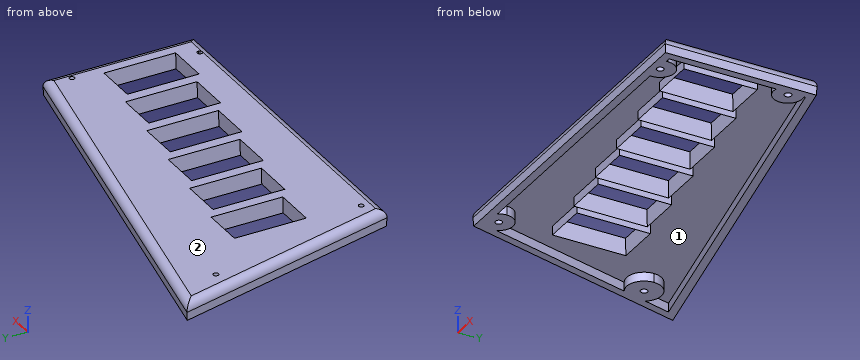
from build123d import *

# Parameters (mm, degrees)
F0_R        = 1.75
F0_W        = 22
F0_H        = 37
F1_DEPTH    = 8.5
F1_TAPER    = -3
F2_DEPTH    = 4.5
F3_T1_DEPTH = 142.1271805444
F3_T3_DEPTH = 228.1816697632
F3_T5_DEPTH = 194.8691049092
F3_T7_DEPTH = 97.8862114568


# Not quite as in the source:
# - a fillet or chamfer that OpenCascade refuses, or shapes differently, is made with other operations: its cross-section is extruded or revolved along the edge and cut away or added


with BuildPart() as f1:
    # F0 (on Top) → F1 (new body)
    with BuildSketch(Plane.XY):
        with BuildLine():
            ThreePointArc((-85.7353818111, -46.3140564233), (-82.1998275149, -55.281625252), (-72.882363358, -52.811342563))
            Line((-72.882363358, -52.811342563), (-84.115426434, -52.811342563))
            Line((-84.115426434, -52.811342563), (-85.7353818111, -46.3140564233))
        make_face()
        with BuildLine():
            Line((-84.115426434, -52.811342563), (-72.882363358, -52.811342563))
            ThreePointArc((-72.882363358, -52.811342563), (-71.9863977223, -50.8998795502), (-71.6790566692, -48.811342563))
            ThreePointArc((-71.6790566692, -48.811342563), (-77.6608605642, -41.6731229923), (-85.7353818111, -46.3140564233))
            Line((-85.7353818111, -46.3140564233), (-84.115426434, -52.811342563))
        make_face()
        with Locations((-78.9290566692, -48.811342563)):
            Circle(F0_R, mode=Mode.SUBTRACT)
        with BuildLine():
            ThreePointArc((73.5070839924, -52.811342563), (72.0709433308, -53.561342563), (70.6348026691, -52.811342563))
            Line((70.6348026691, -52.811342563), (64.8902400226, -52.811342563))
            ThreePointArc((64.8902400226, -52.811342563), (65.5417323383, -54.9628348787), (66.8209433308, -56.811342563))
            Line((66.8209433308, -56.811342563), (77.3209433308, -56.811342563))
            ThreePointArc((77.3209433308, -56.811342563), (78.6001543232, -54.9628348787), (79.2516466389, -52.811342563))
            Line((79.2516466389, -52.811342563), (73.5070839924, -52.811342563))
        make_face()
        with BuildLine():
            ThreePointArc((70.6348026691, -52.811342563), (71.5468947442, -50.1416500527), (73.8209433308, -51.811342563))
            ThreePointArc((73.8209433308, -51.811342563), (73.7406358411, -52.3353911496), (73.5070839924, -52.811342563))
            Line((73.5070839924, -52.811342563), (79.2516466389, -52.811342563))
            ThreePointArc((79.2516466389, -52.811342563), (79.3035984098, -52.3125416331), (79.3209433308, -51.811342563))
            ThreePointArc((79.3209433308, -51.811342563), (71.5697442607, -44.578687484), (64.8902400226, -52.811342563))
            Line((64.8902400226, -52.811342563), (70.6348026691, -52.811342563))
        make_face()
        with BuildLine():
            ThreePointArc((81.75943106, 15.1902968563), (72.6280630891, 8.188657437), (81.75943106, 1.1870180177))
            Line((81.75943106, 1.1870180177), (81.75943106, 15.1902968563))
        make_face()
        with Locations((79.8780630891, 8.188657437)):
            Circle(F0_R, mode=Mode.SUBTRACT)
        with BuildLine():
            Line((81.75943106, 15.1902968563), (81.75943106, 1.1870180177))
            ThreePointArc((81.75943106, 1.1870180177), (83.9978435057, 2.2229295418), (85.75943106, 3.9493165931))
            Line((85.75943106, 3.9493165931), (85.75943106, 12.4279982809))
            ThreePointArc((85.75943106, 12.4279982809), (83.9978435057, 14.1543853322), (81.75943106, 15.1902968563))
        make_face()
        with BuildLine():
            Line((-107.4844802754, 40.9168130189), (-104.4029422618, 28.5574391079))
            ThreePointArc((-104.4029422618, 28.5574391079), (-95.700189339, 28.6381178265), (-91.3719369109, 36.188657437))
            ThreePointArc((-91.3719369109, 36.188657437), (-97.6581749945, 44.5846313066), (-107.4844802754, 40.9168130189))
        make_face()
        with Locations((-100.1219369109, 36.188657437)):
            Circle(F0_R, mode=Mode.SUBTRACT)
        with BuildLine():
            ThreePointArc((-107.4844802754, 40.9168130189), (-108.6120245158, 34.0718408505), (-104.4029422618, 28.5574391079))
            Line((-104.4029422618, 28.5574391079), (-107.4844802754, 40.9168130189))
        make_face()
        with BuildLine():
            ThreePointArc((66.8209433308, -56.811342563), (65.5417323383, -54.9628348787), (64.8902400226, -52.811342563))
            Line((64.8902400226, -52.811342563), (-72.882363358, -52.811342563))
            ThreePointArc((-72.882363358, -52.811342563), (-82.1998275149, -55.281625252), (-85.7353818111, -46.3140564233))
            Line((-85.7353818111, -46.3140564233), (-104.4029422618, 28.5574391079))
            ThreePointArc((-104.4029422618, 28.5574391079), (-108.6120245158, 34.0718408505), (-107.4844802754, 40.9168130189))
            Line((-107.4844802754, 40.9168130189), (-110.8617073408, 54.4621309411))
            Line((-110.8617073408, 54.4621309411), (81.75943106, 15.9099091088))
            Line((81.75943106, 15.9099091088), (81.75943106, 15.1902968563))
            ThreePointArc((81.75943106, 15.1902968563), (83.9978435057, 14.1543853322), (85.75943106, 12.4279982809))
            Line((85.75943106, 12.4279982809), (85.75943106, 19.188657437))
            Line((85.75943106, 19.188657437), (-116.2711964119, 59.6241445901))
            Line((-116.2711964119, 59.6241445901), (-87.24056894, -56.811342563))
            Line((-87.24056894, -56.811342563), (66.8209433308, -56.811342563))
        make_face()
        with BuildLine():
            Line((81.75943106, -52.811342563), (79.2516466389, -52.811342563))
            ThreePointArc((79.2516466389, -52.811342563), (78.6001543232, -54.9628348787), (77.3209433308, -56.811342563))
            Line((77.3209433308, -56.811342563), (85.75943106, -56.811342563))
            Line((85.75943106, -56.811342563), (85.75943106, 3.9493165931))
            ThreePointArc((85.75943106, 3.9493165931), (83.9978435057, 2.2229295418), (81.75943106, 1.1870180177))
            Line((81.75943106, 1.1870180177), (81.75943106, -52.811342563))
        make_face()
        with BuildLine():
            Line((-72.882363358, -52.811342563), (64.8902400226, -52.811342563))
            ThreePointArc((64.8902400226, -52.811342563), (71.5697442607, -44.578687484), (79.3209433308, -51.811342563))
            ThreePointArc((79.3209433308, -51.811342563), (79.3035984098, -52.3125416331), (79.2516466389, -52.811342563))
            Line((79.2516466389, -52.811342563), (81.75943106, -52.811342563))
            Line((81.75943106, -52.811342563), (81.75943106, 1.1870180177))
            ThreePointArc((81.75943106, 1.1870180177), (72.6280630891, 8.188657437), (81.75943106, 15.1902968563))
            Line((81.75943106, 15.1902968563), (81.75943106, 15.9099091088))
            Line((81.75943106, 15.9099091088), (-110.8617073408, 54.4621309411))
            Line((-110.8617073408, 54.4621309411), (-107.4844802754, 40.9168130189))
            ThreePointArc((-107.4844802754, 40.9168130189), (-97.6581749945, 44.5846313066), (-91.3719369109, 36.188657437))
            ThreePointArc((-91.3719369109, 36.188657437), (-95.700189339, 28.6381178265), (-104.4029422618, 28.5574391079))
            Line((-104.4029422618, 28.5574391079), (-85.7353818111, -46.3140564233))
            ThreePointArc((-85.7353818111, -46.3140564233), (-77.6608605642, -41.6731229923), (-71.6790566692, -48.811342563))
            ThreePointArc((-71.6790566692, -48.811342563), (-71.9863977223, -50.8998795502), (-72.882363358, -52.811342563))
        make_face()
        with Locations((-66.1195590496, -4.311342563)):
            Rectangle(F0_W, F0_H, mode=Mode.SUBTRACT)
        with Locations((-39.6195590496, -8.311342563)):
            Rectangle(F0_W, F0_H, mode=Mode.SUBTRACT)
        with Locations((13.3804409504, -16.311342563)):
            Rectangle(F0_W, F0_H, mode=Mode.SUBTRACT)
        with Locations((-13.1195590496, -12.311342563)):
            Rectangle(F0_W, F0_H, mode=Mode.SUBTRACT)
        with Locations((39.8804409504, -20.311342563)):
            Rectangle(F0_W, F0_H, mode=Mode.SUBTRACT)
        with Locations((66.3804409504, -24.311342563)):
            Rectangle(F0_W, F0_H, mode=Mode.SUBTRACT)
    extrude(amount=F1_DEPTH, taper=F1_TAPER)

    # F0 (on Top) → F2 (cut)
    with BuildSketch(Plane.XY):
        with BuildLine():
            Line((-72.882363358, -52.811342563), (64.8902400226, -52.811342563))
            ThreePointArc((64.8902400226, -52.811342563), (71.5697442607, -44.578687484), (79.3209433308, -51.811342563))
            ThreePointArc((79.3209433308, -51.811342563), (79.3035984098, -52.3125416331), (79.2516466389, -52.811342563))
            Line((79.2516466389, -52.811342563), (81.75943106, -52.811342563))
            Line((81.75943106, -52.811342563), (81.75943106, 1.1870180177))
            ThreePointArc((81.75943106, 1.1870180177), (72.6280630891, 8.188657437), (81.75943106, 15.1902968563))
            Line((81.75943106, 15.1902968563), (81.75943106, 15.9099091088))
            Line((81.75943106, 15.9099091088), (-110.8617073408, 54.4621309411))
            Line((-110.8617073408, 54.4621309411), (-107.4844802754, 40.9168130189))
            ThreePointArc((-107.4844802754, 40.9168130189), (-97.6581749945, 44.5846313066), (-91.3719369109, 36.188657437))
            ThreePointArc((-91.3719369109, 36.188657437), (-95.700189339, 28.6381178265), (-104.4029422618, 28.5574391079))
            Line((-104.4029422618, 28.5574391079), (-85.7353818111, -46.3140564233))
            ThreePointArc((-85.7353818111, -46.3140564233), (-77.6608605642, -41.6731229923), (-71.6790566692, -48.811342563))
            ThreePointArc((-71.6790566692, -48.811342563), (-71.9863977223, -50.8998795502), (-72.882363358, -52.811342563))
        make_face()
        with Locations((-66.1195590496, -4.311342563)):
            Rectangle(F0_W, F0_H, mode=Mode.SUBTRACT)
        with Locations((-39.6195590496, -8.311342563)):
            Rectangle(F0_W, F0_H, mode=Mode.SUBTRACT)
        with Locations((13.3804409504, -16.311342563)):
            Rectangle(F0_W, F0_H, mode=Mode.SUBTRACT)
        with Locations((-13.1195590496, -12.311342563)):
            Rectangle(F0_W, F0_H, mode=Mode.SUBTRACT)
        with Locations((39.8804409504, -20.311342563)):
            Rectangle(F0_W, F0_H, mode=Mode.SUBTRACT)
        with Locations((66.3804409504, -24.311342563)):
            Rectangle(F0_W, F0_H, mode=Mode.SUBTRACT)
    extrude(amount=F2_DEPTH, mode=Mode.SUBTRACT)

    # F3: fillet of radius 4 on 4 edges, made by hand

    # F3_s2 → F3_t1 (cut)
    with BuildSketch(Plane(origin=(-23.5203588914, 94.3350069914, 0), x_dir=(0, 0, 1), z_dir=(0.2419218956, -0.9702957263, 0))):
        with BuildLine():
            ThreePointArc((4.290656175, 98.6179226466), (7.2534183028, 97.5249019916), (8.5, 94.6234045075))
            Line((8.5, 94.6234045075), (8.5, 98.8385250087))
            Line((8.5, 98.8385250087), (4.290656175, 98.6179226466))
        make_face()
    extrude(amount=F3_T1_DEPTH, mode=Mode.SUBTRACT)

    # F3_s4 → F3_t3 (cut)
    with BuildSketch(Plane(origin=(89.4546965917, -17.9039400119, 0), x_dir=(0, 0, 1), z_dir=(-0.980553261, 0.1962531587, 0))):
        with BuildLine():
            ThreePointArc((4.290656175, 35.8709236176), (7.2534183028, 34.7779029626), (8.5, 31.8764054785))
            Line((8.5, 31.8764054785), (8.5, 36.0915259797))
            Line((8.5, 36.0915259797), (4.290656175, 35.8709236176))
        make_face()
    extrude(amount=F3_T3_DEPTH, mode=Mode.SUBTRACT)

    # F3_s6 → F3_t5 (cut)
    with BuildSketch(Plane.YZ.offset(-98.1264064725)):
        with BuildLine():
            ThreePointArc((-53.0416881858, 8.5), (-55.9431856699, 7.2534183028), (-57.0362063248, 4.290656175))
            Line((-57.0362063248, 4.290656175), (-57.2568086869, 8.5))
            Line((-57.2568086869, 8.5), (-53.0416881858, 8.5))
        make_face()
    extrude(amount=F3_T5_DEPTH, mode=Mode.SUBTRACT)

    # F3_s8 → F3_t7 (cut)
    with BuildSketch(Plane.XZ.offset(-30.091601517)):
        with BuildLine():
            ThreePointArc((81.9897766828, 8.5), (84.8912741668, 7.2534183028), (85.9842948218, 4.290656175))
            Line((85.9842948218, 4.290656175), (86.2048971839, 8.5))
            Line((86.2048971839, 8.5), (81.9897766828, 8.5))
        make_face()
    extrude(amount=F3_T7_DEPTH, mode=Mode.SUBTRACT)


solid = f1.part
Verification items for the finished model (mm, model axes). Face numbers are marked on the shaded views. Give positions to 0.01 mm unless a question says otherwise; leave off trailing zeros.
1) Thickness scan on line 1 along Y through (x, z) = (-7, 3.75); line 2 along Z through (x, y) = (-75.5, -42); line 3 along X through (y, z) = (-2, 5.5). Record the ranges inside material, lowest first.
2) Depth check by flat-ended pin: pin 1 Ø3.5 at (y, z) = (-18, 1.5) entering from -X; pin 2 Ø1 at (y, z) = (-12.5, 2) entering from +X; pin 3 Ø1 at (x, y) = (-10, 25) entering from -Z. Enter the tip coordinate at first touch or a pass-through.
3) Sectioned sample at A-A, the plane z = 1.5. Count the separate pieces of the cut face and the enclosed holes in it, then the cut area to 3 significant figures.
4) Draft check along X on the marked faces 1 and 2. Enter one of: pulls with the +X half, pulls with the -X half, needs draft (parallel to the pull), parting line crosses it, or undercut.
Answers:
1. line 1: y = -57.01 to -52.81, -30.81 to -30.61, 5.99 to 6.19, 33.67 to 37.95
1. line 2: z = 4.5 to 8.5
1. line 3: x = -101.01 to -76.83, -55.41 to -50.33, -28.91 to -23.83, -2.41 to 2.67, 24.09 to 85.86
2. pin 1: stops at x = -97.44
2. pin 2: stops at x = 85.89
2. pin 3: stops at z = 4.5
3. separate pieces: 7
3. enclosed holes: 11
3. area: 2,850 mm2
4. face 1: undercut
4. face 2: needs draft
